from build123d import *

# Parameters (mm, degrees)
SKETCH2_W           = 90
SKETCH2_H           = 5
BOSS_EXTRUDE1_DEPTH = 21
SKETCH3_W           = 90
SKETCH3_H           = 5
BOSS_EXTRUDE2_DEPTH = 105
FILLET1_R           = 10
SKETCH4_R           = 4.025
CUT_EXTRUDE1_DEPTH  = 118.631840928
CUT_EXTRUDE2_DEPTH  = 119.415581745
CUT_EXTRUDE3_DEPTH  = 10


with BuildPart() as part:
    # Sketch2 → Boss-Extrude1 (new body)
    with BuildSketch(Plane.XY):
        Rectangle(SKETCH2_W, SKETCH2_H)
    extrude(amount=BOSS_EXTRUDE1_DEPTH)

    # Sketch3 → Boss-Extrude2 (add)
    with BuildSketch(Plane(origin=(0, 2.5, 0), x_dir=(1, 0, 0), z_dir=(0, 1, 0))):
        with Locations((0, -2.5)):
            Rectangle(SKETCH3_W, SKETCH3_H)
    extrude(amount=BOSS_EXTRUDE2_DEPTH)

    # Fillet1
    fillet1_edges = [part.edges().sort_by_distance(p)[0] for p in [
        (45, 107.5, 2.5),
    ]]
    fillet(fillet1_edges, radius=FILLET1_R)

    # Sketch4 → Cut-Extrude1 (cut, through all)
    with BuildSketch(Plane.XY.offset(5)):
        with Locations((33, 95.5)):
            Circle(SKETCH4_R)
    extrude(amount=-CUT_EXTRUDE1_DEPTH, mode=Mode.SUBTRACT)

    # Sketch6 → Cut-Extrude2 (cut, through all)
    with BuildSketch(Plane.XY.offset(21)):
        Polygon((45, 77.5), (15, -2.5), (45, -2.5), align=None)
        Polygon((-45, 27.5), (-15, 107.5), (-45, 107.5), align=None)
    extrude(amount=-CUT_EXTRUDE2_DEPTH, mode=Mode.SUBTRACT)

    # Sketch7 → Cut-Extrude3 (cut)
    with BuildSketch(Plane(origin=(0, 2.5, 0), x_dir=(1, 0, 0), z_dir=(0, 1, 0))):
        with BuildLine():
            Line((6.875, -15.35), (-35, -15.35))
            ThreePointArc((-35, -15.35), (-36.6, -13.75), (-35, -12.15))
            Line((-35, -12.15), (6.875, -12.15))
            ThreePointArc((6.875, -12.15), (8.475, -13.75), (6.875, -15.35))
        make_face()
    extrude(amount=-CUT_EXTRUDE3_DEPTH, mode=Mode.SUBTRACT)


solid = part.part
Read the model definition and answer for the solid it produces. Units are mm, in the model's axes. A direction names the side the tool comes from. Coordinates: 2 decimals unless noted, no trailing zeros. Order: outer loops, then holes, each group sorted by start corner. A loop starts at its lowest first (then second) coordinate and runs counter-clockwise, first axis right, second up. Notation, with made-up numbers: M 59,63 L 87,63 A7 cw 87,74 Z; hole C -38,-39 d6. An arc over 180 degrees is marked long. Put each result on its own line as item: value. Start each with the question number.
Item 1: Section B-B, the plane z = 13.75 is taken. Determine the outline of the cut face in (x, y) (3 decimals).
Item 2: Section C-C, the plane x = 1.5 is taken. Determine the outline of the cut face in (y, z).
Item 3: Consider probe 1 along Y at (x, z) = (-9, 11.25); probe 2 along Z at (x, y) = (-25.5, 50); probe 3 along X at (y, z) = (3, 2). Determine where each line is inside the solid, lowest interval first. Write a range as [from, to].
Item 4: Section D-D, the plane y = 23.5 is taken. Determine the outline of the cut face in (x, z).
Item 5: Given pin 1 Ø4 at (x, y) = (26, 72) entering from +Z, flat-ended and moving along its own axis, determine where the tip first touches the part or whether it passes through.
Item 6: The mould has two halves that part along Z. Classify faces 1 (the face through (-36.6, 0, 13.8)), 2 (the face through (45, 87, 3)), 3 (the face through (-1, 52, 0)): +Z half, -Z half, draft (parallel to the pull), parting line (faces both ways), or undercut.
Item 7: Section A-A, the plane y = 95.5 is taken. Determine the outline of the cut face in (x, z) (3 decimals), plus the area to 3 significant figures.
Item 8: For faces 4 (the face through (10, 107.5, 2)), 5 (the face through (-1, 54, 5)), 6 (the face through (8.475, 0.035, 13.715)), determine the directions among +Z, -Z, +X, -X, +Y, -Y from which every point of the face is accessible in a straight line to the end or side of a thin tool.
Computed:
1. outline: M -45,-2.5 L -36.6,-2.5 L -36.6,2.5 L -45,2.5 Z; M 8.475,-2.5 L 15,-2.5 L 16.875,2.5 L 8.475,2.5 Z
2. outline: M -2.5,0 L 107.5,0 L 107.5,5 L 2.5,5 L 2.5,12.15 L -2.5,12.15 Z; M -2.5,15.35 L 2.5,15.35 L 2.5,21 L -2.5,21 Z
3. probe 1: y = [-2.5, 2.5]
3. probe 2: z = [0, 5]
3. probe 3: x = [-45, 17.06]
4. outline: M -45,0 L 24.75,0 L 24.75,5 L -45,5 Z
5. pin 1: stops at z = 5
6. face 1: undercut
6. face 2: draft
6. face 3: -Z half
7. outline: M -19.5,0 L 28.975,0 L 28.975,5 L -19.5,5 Z; M 37.025,0 L 45,0 L 45,5 L 37.025,5 Z
7. area: 282 mm2
8. face 4: +Z, -Z, +X, -X, +Y
8. face 5: +Z, +X, -X, +Y
8. face 6: +Y, -Y
